Job drawing, mm, ordinate dimensions from the low corner. One solid piece. A direction names the side the tool comes from. Round coordinates to 2 decimals unless told otherwise and drop trailing zeros. Order: outer loops, then holes, each group sorted by start corner. A loop starts at its lowest first (then second) coordinate and runs counter-clockwise, first axis right, second up. Notation, with made-up numbers: (87, 15.5) -> (108, 15.5) arc R18 ccw to (108, 49.5) -> close; hole circle Ø9 at (61, -23). An arc over 180 degrees is marked (long way). Answer as a JSON object with one key per item and string values. Group by question number.
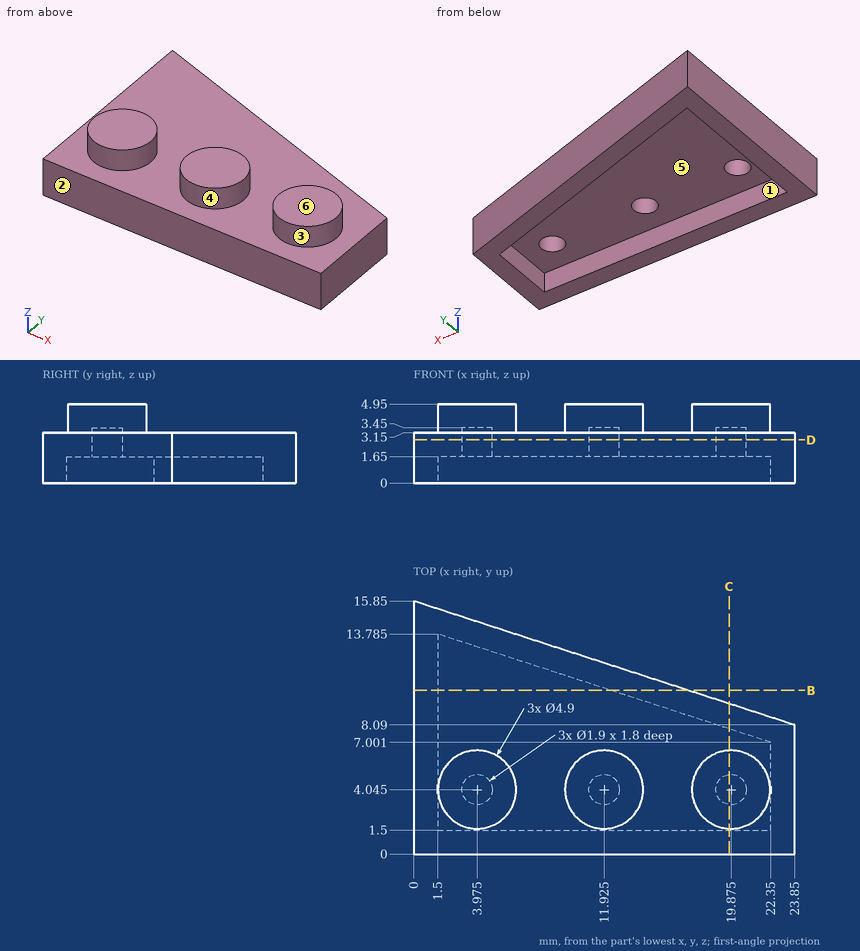
Q1. Wall check: line 1 (X direction, y = 4, z = 4.5) (1 decimal); line 2 (X direction, y = 4.75, z = 0.65); line 3 (Z direction, x = 3.5, y = 7.5). Give the ranges that are in metal, low to high. Write a range as [from, to].
Q2. Which spindle directions (+Z, -Z, +X, -X, +Y, -Y) get a long thin tool onto all of the face, cutting with end or side? Do the marked faces 1, 2 and 3. Say none if no direction does.
Q3. Band-saw the part on D-D (z = 2.7). Count the separate pieces of the cut face and the enclosed holes in it, plus the area to 3 significant figures.
Q4. Band-saw the part on B-B (y = 10.25). List the corners of the cut face in (x, z), plus the area to 3 significant figures.
Q5. Two-plate mould, pull along Y, no slides. Class the marked faces 4, 5 and 6: +Y half, -Y half, draft (parallel to the pull), parting line (faces both ways), or undercut.
Q6. Drop flat-ended pins along their axis: pin 1 Ø1.8 at (x, z) = (8, 1) entering from +Y; pin 2 Ø2 at (x, y) = (12, 4.5) entering from -Z; pin 3 Ø1.5 at (x, y) = (3.975, 4.045) entering from -Z; pin 4 Ø2 at (x, y) = (12.5, 14) entering from -Z. Give the stop position or say it passes through.
Q7. Band-saw the part on C-C (x = 19.75). List the corners of the cut face in (y, z).
Completed:
{
 "1": {"line 1": "[1.5, 6.4], [9.5, 14.4], [17.4, 22.3]", "line 2": "[0, 1.5], [22.35, 23.85]", "line 3": "[1.65, 3.15]"},
 "2": {"face 1": "-Z", "face 2": "+Z, -Z, +X, -X, -Y", "face 3": "+Z"},
 "3": {"separate pieces": "1", "enclosed holes": "3", "area": "277 mm2"},
 "4": {"outline": "(0, 0) -> (1.5, 0) -> (1.5, 1.65) -> (12.36, 1.65) -> (12.36, 0) -> (17.21, 0) -> (17.21, 3.15) -> (0, 3.15) -> close", "area": "36.3 mm2"},
 "5": {"face 4": "parting line", "face 5": "undercut", "face 6": "draft"},
 "6": {"pin 1": "y = 13.54", "pin 2": "z = 1.65", "pin 3": "z = 3.45", "pin 4": "through"},
 "7": {"outline": "(0, 0) -> (1.5, 0) -> (1.5, 1.65) -> (3.1, 1.65) -> (3.1, 3.45) -> (4.99, 3.45) -> (4.99, 1.65) -> (7.85, 1.65) -> (7.85, 0) -> (9.42, 0) -> (9.42, 3.15) -> (6.49, 3.15) -> (6.49, 4.95) -> (1.6, 4.95) -> (1.6, 3.15) -> (0, 3.15) -> close"}
}
